Design review of the part built by this model. Coordinates are the model's own, in mm. Face numbers are marked on the shaded views. A direction names the side the tool comes from. Coordinates: 2 decimals unless noted, no trailing zeros. Write each loop counter-clockwise with the first axis right and the second up, starting at its lowest first coordinate (ties: lowest second). Pieces come first, ordered by that corner, then holes. Notation, with made-up numbers: (50.25, 60) - (67.25, 60) arc R23 ccw to (67.25, 98) - close; hole circle Ø11 at (60.25, -38.75). An arc over 180 degrees is marked (long way). Use a Markdown table: item, result.
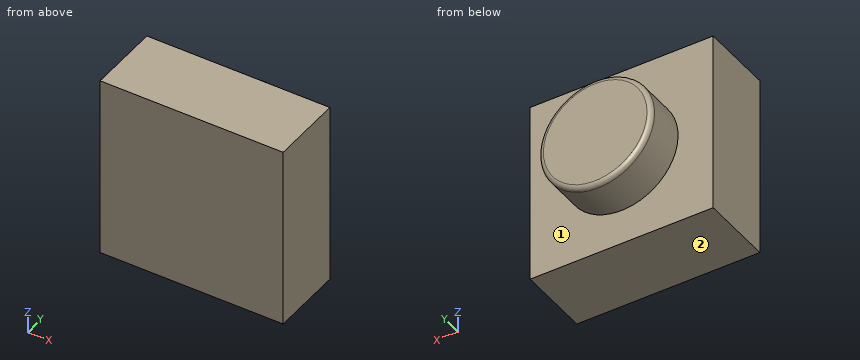
from build123d import *

# Parameters (mm, degrees)
SKETCH_1_W      = 7.95
SKETCH_1_H      = 7.95
EXTRUDE_1_DEPTH = 3.18
SKETCH_2_R      = 2.45
EXTRUDE_2_DEPTH = 1.8
FILLET_1_R      = 0.2


with BuildPart() as part:
    # 草图1 → 凸台-拉伸1 (new body)
    with BuildSketch(Plane(origin=(0, 0, 0), x_dir=(1, 0, 0), z_dir=(0, 1, 0))):
        with Locations((27.642590822, 13.353871893)):
            Rectangle(SKETCH_1_W, SKETCH_1_H)
    extrude(amount=EXTRUDE_1_DEPTH)

    # 草图2 → 凸台-拉伸2 (add)
    with BuildSketch(Plane(origin=(0, 3.18, 0), x_dir=(1, 0, 0), z_dir=(0, 1, 0))):
        with Locations(Location((27.642590822, 13.353871893, 0), (0, 0, 270))):
            Circle(SKETCH_2_R)
    extrude(amount=EXTRUDE_2_DEPTH)

    # 圆角1
    fillet_1_edges = [part.edges().sort_by_distance(p)[0] for p in [
        (27.642590822, 4.98, -15.803871893),
    ]]
    fillet(fillet_1_edges, radius=FILLET_1_R)


solid = part.part
(1) Machinability: for the marked faces 1 and 2, which of the approach directions +Z, -Z, +X, -X, +Y, -Y give a long, thin tool a straight path to every point of the face, cutting with its end or side? Answer none if there is none.
Determined:
| item | result |
|---|---|
| face 1 | +Y |
| face 2 | -Z, +X, -X, +Y, -Y |
(2) Take a section at C-C on y = 4.35. Write out the cut boundary in (x, z).
Determined:
| item | result |
|---|---|
| outline | circle Ø4.9 at (27.64, -13.35) |
(3) For pin 1 (2 mm diameter, centred on x = 28, y = 3.5, fed in from -Z), flat-tipped, find the tip position at first contact; note if it passes through.
Determined:
| item | result |
|---|---|
| pin 1 | z = -17.33 |
(4) Take a section at A-A on x = 30.75. Write out the cut boundary in (y, z), and give its area (3 significant figures).
Determined:
| item | result |
|---|---|
| outline | (0, -17.33) - (3.18, -17.33) - (3.18, -9.38) - (0, -9.38) - close |
| area | 25.3 mm2 |
(5) For L1, parallel to Y at x = 31.25, z = -13.5; L2, parallel to X at y = 4.15, z = -11.5; L3, parallel to Y at x = 28.5, z = -15.5, list the stretches that pass through material, from the lowest coordinate up. Write a range as from..to.
Determined:
| item | result |
|---|---|
| L1 | 0..3.18 |
| L2 | 26.04..29.24 |
| L3 | 0..4.97 |
(6) Take a section at B-B on z = -16. Write out the cut boundary in (x, y), and give its area (3 significant figures).
Determined:
| item | result |
|---|---|
| outline | (23.67, 0) - (31.62, 0) - (31.62, 3.18) - (23.67, 3.18) - close |
| area | 25.3 mm2 |
